Geometry: final body of the model. Coordinates: model frame, mm. Face numbers are marked on the shaded views. A direction names the side the tool comes from. Coordinates: 2 decimals unless noted, no trailing zeros. Order: outer loops, then holes, each group sorted by start corner. A loop starts at its lowest first (then second) coordinate and runs counter-clockwise, first axis right, second up. Notation, with made-up numbers: M 60,-10.75 L 78,-10.75 A28 ccw 78,20.25 Z; hole C 48.25,69.5 d11. An arc over 180 degrees is marked long. One line per question, with ' | ' between items.
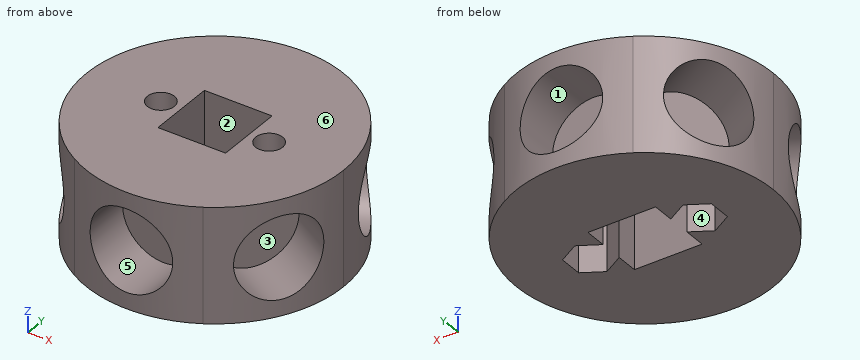
from build123d import *

# Parameters (mm, degrees)
F1_DEPTH  = 17
F5_R      = 6.1
F6_DEPTH  = 9
F7_COUNT  = 6
F9_D      = 4
F10_R     = 2
F11_DEPTH = 10
F12_DEPTH = 17.0010001


with BuildPart() as f1:
    # F0 (on Top) → F1 (new body)
    with BuildSketch(Plane.XY):
        with BuildLine():
            Line((0, 0), (9.5, 16.4544826719))
            ThreePointArc((9.5, 16.4544826719), (0, 19), (-9.5, 16.4544826719))
            Line((-9.5, 16.4544826719), (0, 0))
        make_face()
    extrude(amount=F1_DEPTH)

    # F5 (on offset) → F6 (cut)
    with BuildSketch(Plane.XZ.offset(-20)):
        with Locations((0, 8.5)):
            Circle(F5_R)
    extrude(amount=F6_DEPTH, mode=Mode.SUBTRACT)

    # F7: F1 ×6 about axis
    f7_axis = Axis((0, 0, 0), (0, 0, 1))


with BuildPart() as f1_1:
    add(f1.part)
    for i in range(1, F7_COUNT):
        add(f1.part.rotate(f7_axis, i * 360 / F7_COUNT))

    # F9 (through all)
    with Locations(Plane(origin=(0, 0, 0), x_dir=(1, 0, 0), z_dir=(0, 0, -1))):
        with Locations((-8, 0), (8, 0)):
            Hole(F9_D / 2)

    # F10 (on face) → F11 (cut)
    with BuildSketch(Plane(origin=(0, 0, 0), x_dir=(1, 0, 0), z_dir=(0, 0, -1))):
        Polygon((-5, -1.7320508076), (-5, 1.7320508076), (-8, 3.4641016151), (-11, 1.7320508076), (-11, -1.7320508076), (-8, -3.4641016151), align=None)
        with Locations((-8, 0)):
            Circle(F10_R, mode=Mode.SUBTRACT)
        Polygon((5, 1.7320508076), (5, -1.7320508076), (8, -3.4641016151), (11, -1.7320508076), (11, 1.7320508076), (8, 3.4641016151), align=None)
        with Locations((8, 0)):
            Circle(F10_R, mode=Mode.SUBTRACT)
    extrude(amount=-F11_DEPTH, mode=Mode.SUBTRACT)

    # F8 (on face) → F12 (cut, through all)
    with BuildSketch(Plane(origin=(0, 0, 0), x_dir=(1, 0, 0), z_dir=(0, 0, -1))):
        with BuildLine():
            Line((0, 2.1), (0, 5))
            Line((0, 5), (-5, 5))
            Line((-5, 5), (-5, -5))
            Line((-5, -5), (5, -5))
            Line((5, -5), (5, 5))
            Line((5, 5), (2.8867513459, 5))
            Line((2.8867513459, 5), (1.05, 1.8186533479))
            ThreePointArc((1.05, 1.8186533479), (1.0751032483, 1.8039271065), (1.1, 1.788854382))
            ThreePointArc((1.1, 1.788854382), (1.833030278, 1.0246950766), (2.1, 0))
            ThreePointArc((2.1, 0), (1.833030278, -1.0246950766), (1.1, -1.788854382))
            ThreePointArc((1.1, -1.788854382), (0, -2.1), (-1.1, -1.788854382))
            ThreePointArc((-1.1, -1.788854382), (-2.1, 0), (-1.1, 1.788854382))
            ThreePointArc((-1.1, 1.788854382), (-0.5715793024, 2.020716977), (0, 2.1))
        make_face()
        with BuildLine():
            Line((2.8867513459, 5), (0, 5))
            Line((0, 5), (0, 2.1))
            ThreePointArc((0, 2.1), (0.5435199947, 2.0284442352), (1.05, 1.8186533479))
            Line((1.05, 1.8186533479), (2.8867513459, 5))
        make_face()
        with BuildLine():
            Line((0, 0), (0, 2.1))
            ThreePointArc((0, 2.1), (-0.5715793024, 2.020716977), (-1.1, 1.788854382))
            Line((-1.1, 1.788854382), (-1.1, -1.788854382))
            ThreePointArc((-1.1, -1.788854382), (0, -2.1), (1.1, -1.788854382))
            Line((1.1, -1.788854382), (1.1, 1.788854382))
            ThreePointArc((1.1, 1.788854382), (1.0751032483, 1.8039271065), (1.05, 1.8186533479))
            Line((1.05, 1.8186533479), (0, 0))
        make_face()
        with BuildLine():
            Line((-1.1, -1.788854382), (-1.1, 1.788854382))
            ThreePointArc((-1.1, 1.788854382), (-2.1, 0), (-1.1, -1.788854382))
        make_face()
        with BuildLine():
            ThreePointArc((2.1, 0), (1.833030278, 1.0246950766), (1.1, 1.788854382))
            Line((1.1, 1.788854382), (1.1, -1.788854382))
            ThreePointArc((1.1, -1.788854382), (1.833030278, -1.0246950766), (2.1, 0))
        make_face()
        with BuildLine():
            ThreePointArc((1.05, 1.8186533479), (0.5435199947, 2.0284442352), (0, 2.1))
            Line((0, 2.1), (0, 0))
            Line((0, 0), (1.05, 1.8186533479))
        make_face()
    extrude(amount=-F12_DEPTH, mode=Mode.SUBTRACT)


solid = f1_1.part
1. Draft query along X for the marked faces 5 and 6. Return one class per face: pulls with the +X half, pulls with the -X half, needs draft (parallel to the pull), parting line crosses it, or undercut.
Response values:
face 5: undercut | face 6: needs draft
2. Section B-B, the plane y = -1. Give the number of separate pieces and of enclosed holes in the cut face, and give its area (3 significant figures).
Response values:
separate pieces: 4 | enclosed holes: 2 | area: 291 mm^2
3. Section C-C, the plane y = 16. Output: boundary loops of the cut face in (x, z), and give its area (3 significant figures).
Response values:
outline: M -10.25,0 L 10.25,0 L 10.25,17 L -10.25,17 Z; hole C 0,8.5 d12.2 | area: 231 mm^2
4. Section A-A, the plane x = 0. Output: boundary loops of the cut face in (y, z), and give its area (3 significant figures).
Response values:
outline: M -19,0 L -5,0 L -5,17 L -19,17 L -19,14.6 L -11,14.6 L -11,2.4 L -19,2.4 Z; M 5,0 L 19,0 L 19,2.4 L 11,2.4 L 11,14.6 L 19,14.6 L 19,17 L 5,17 Z | area: 281 mm^2
5. Access query for the marked faces 1, 2, 3 and 4. Directions: +Z, -Z, +X, -X, +Y, -Y. A direction counts if a zero-diameter tool reaches every point of the face in a straight line with its end or side. Return the directions, or none.
Response values:
face 1: +Y | face 2: +Z, -Z | face 3: none | face 4: -Z
6. Pin query (flat end, axial travel): P1, Ø2, axis at y = 7, z = 4, coming from the -X side; P2, Ø2, axis at x = 9, z = 2, coming from the +Y side; P3, Ø3.5, axis at x = -1, z = 9, coming from the -Y side; P4, Ø3, axis at x = -7, y = -1.5, coming from the -Z side. Return the tip coordinate at first contact, or that it passes through.
Response values:
P1: stops at x = -18.01 | P2: stops at y = 17.23 | P3: stops at y = -11 | P4: stops at z = 0
7. Material intervals for line 1 (Y direction, x = -3, z = 8); line 2 (Z direction, x = 0, y = -13); line 3 (Y direction, x = 10.5, z = 11.25), sorted ascending. Write a range as [from, to].
Response values:
line 1: y = [-11, -5], [5, 11] | line 2: z = [0, 2.4], [14.6, 17] | line 3: y = [-15.84, -12.35], [-3.81, 3.81], [12.35, 15.84]
